```python
from build123d import *

# Parameters (mm, degrees)
CORTAR_EXTRUIR1_DEPTH = 11
CORTAR_EXTRUIR2_DEPTH = 10


with BuildPart() as part:
    # Croquis1 → Revolución1 (revolve)
    with BuildSketch(Plane(origin=(0, 0, 0), x_dir=(0, 0, -1), z_dir=(1, 0, 0))):
        with BuildLine():
            Line((0, 0), (0, 10.5))
            Line((0, 10.5), (0.75, 10.5))
            ThreePointArc((0.75, 10.5), (2.25, 9), (3.75, 10.5))
            Line((3.75, 10.5), (4.5, 10.5))
            Line((4.5, 10.5), (4.5, 3.5))
            Line((4.5, 3.5), (10, 3.5))
            Line((10, 3.5), (10, 0))
            Line((10, 0), (0, 0))
        make_face()
    revolve(axis=Axis((0, 0, 0), (0, 0, -1)))

    # Croquis2 → Cortar-Extruir1 (cut, through all)
    with BuildSketch(Plane(origin=(0, 0, -10), x_dir=(-1, 0, 0), z_dir=(0, 0, -1))):
        with BuildLine():
            Line((-1.161895004, 1.1), (1.161895004, 1.1))
            ThreePointArc((1.161895004, 1.1), (0, -1.6), (-1.161895004, 1.1))
        make_face()
    extrude(amount=-CORTAR_EXTRUIR1_DEPTH, mode=Mode.SUBTRACT)

    # Croquis3 → Cortar-Extruir2 (cut)
    with BuildSketch(Plane(origin=(0, 0, -10), x_dir=(-1, 0, 0), z_dir=(0, 0, -1))):
        with BuildLine():
            Line((-1.183215957, 1.15), (1.183215957, 1.15))
            ThreePointArc((1.183215957, 1.15), (0, -1.65), (-1.183215957, 1.15))
        make_face()
    extrude(amount=-CORTAR_EXTRUIR2_DEPTH, mode=Mode.SUBTRACT)


solid = part.part
```
Build history of the part. All positions in model axes, mm. A direction names the side the tool comes from. Give positions to 0.01 mm unless a question says otherwise; leave off trailing zeros. Loops run counter-clockwise (first coordinate to the right, second up) from the corner with the lowest first, then second, coordinate; pieces in that order, holes last.
1) Band-saw the part on B-B on y = 0. List the corners of the cut face in (x, z).
Values follow:
outline: (-10.5, -4.5) - (-3.5, -4.5) - (-3.5, -10) - (-1.65, -10) - (-1.65, 0) - (-10.5, 0) - (-10.5, -0.75) arc R1.5 cw to (-10.5, -3.75) - close; (1.65, -10) - (3.5, -10) - (3.5, -4.5) - (10.5, -4.5) - (10.5, -3.75) arc R1.5 cw to (10.5, -0.75) - (10.5, 0) - (1.65, 0) - close
2) 3-axis set-ups, long thin cutter, end or side, ignore diameter. For faces 1 (the face through (3.2, 10, -4.1)), 2 (the face through (0, 5, -4.5)): which of +Z, -Z, +X, -X, +Y, -Y reach the whole face in a straight line?
Values follow:
face 1: +Z, -Z
face 2: -Z
3) Drop flat-ended pins along their axis: P1, Ø2.5, axis at x = 0, y = 0, coming from the -Z side; P2, Ø5, axis at x = 8, y = 7.5, coming from the -Z side; P3, Ø2.5, axis at x = 0, z = -6.5, coming from the -Y side; P4, Ø1, axis at y = 8, z = -4.5, coming from the +X side. Give the stop position or say it passes through.
Values follow:
P1: stops at z = -10
P2: stops at z = -4.5
P3: stops at y = -3.5
P4: stops at x = 7.35
4) Probe line 1 along X through (y, z) = (0, -7.5); line 2 along Y through (x, z) = (1, -6.5); line 3 along Z through (x, y) = (-0.25, -4.75). List the from-to ranges inside material, lowest first.
Values follow:
line 1: x = -3.5 to -1.65, 1.65 to 3.5
line 2: y = -3.35 to -1.31, 1.15 to 3.35
line 3: z = -4.5 to 0
5) Two-plate mould, pull along X, no slides. Class faces 3 (the face through (3.2, 10, -0.4)), 4 (the face through (0, 1.15, -5)), 5 (the face through (0, 2, -10)): released by +X, released by -X, zero draft, split by the parting line, or undercut.
Values follow:
face 3: split by the parting line
face 4: undercut
face 5: zero draft
6) Band-saw the part on A-A on x = 0. List the corners of the cut face in (y, z).
Values follow:
outline: (-10.5, -4.5) - (-3.5, -4.5) - (-3.5, -10) - (-1.65, -10) - (-1.65, 0) - (-10.5, 0) - (-10.5, -0.75) arc R1.5 cw to (-10.5, -3.75) - close; (1.15, -10) - (3.5, -10) - (3.5, -4.5) - (10.5, -4.5) - (10.5, -3.75) arc R1.5 cw to (10.5, -0.75) - (10.5, 0) - (1.15, 0) - close
7) Band-saw the part on C-C on z = -6. List the corners of the cut face in (x, y), then the cut area to 3 significant figures.
Values follow:
outline: circle Ø7 at (0, 0); hole (-1.18, 1.15) arc R1.65 ccw (long way) to (1.18, 1.15) - close
area: 30.7 mm2
